```python
from build123d import *

# Parameters (mm, degrees)
F1_DEPTH = 3
F2_DEPTH = 30
F3_W     = 20
F3_H     = 10
F4_DEPTH = 35


with BuildPart() as f1:
    # F0 (on Front) → F1 (new body)
    with BuildSketch(Plane.XZ):
        Polygon((0, 40), (0, 0), (30, 0), (30, 10), (20, 10), (10, 40), align=None)
    extrude(amount=F1_DEPTH)

    # F1_face (on face) → F2 (join)
    with BuildSketch(Plane(origin=(10.666667, -3, 16), x_dir=(1, 0, 0), z_dir=(0, -1, 0))):
        Polygon((-10.666667, 24), (-10.666667, -16), (19.333333, -16), (19.333333, -6), (9.333333, -6), (-0.666667, 24), align=None)
    extrude(amount=F2_DEPTH)

    # F3 (on face) → F4 (cut)
    with BuildSketch(Plane.XY.offset(40)):
        with Locations((20, -15)):
            Rectangle(F3_W, F3_H)
    extrude(amount=-F4_DEPTH, mode=Mode.SUBTRACT)


solid = f1.part
```
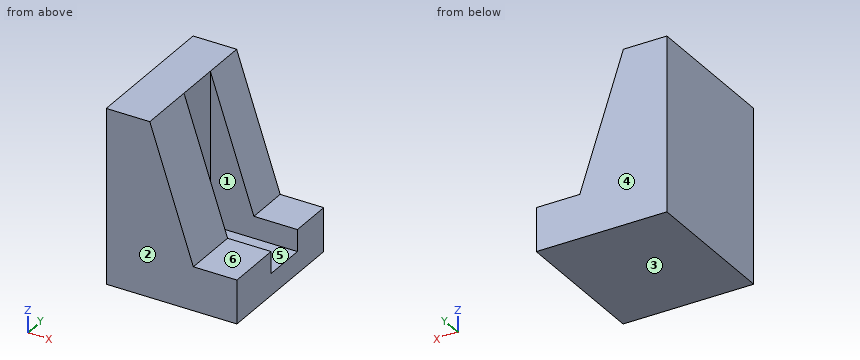
Can you work these out from the model? Positions are in its coordinate system, mm. Face numbers are marked on the shaded views. A direction names the side the tool comes from. Coordinates: 2 decimals unless noted, no trailing zeros. Loops run counter-clockwise (first coordinate to the right, second up) from the corner with the lowest first, then second, coordinate; pieces in that order, holes last. Notation, with made-up numbers: (-16, 27.5) -> (34, 27.5) arc R7 ccw to (34, 34.5) -> close; hole circle Ø1 at (11.25, -28). An arc over 180 degrees is marked (long way). Put each result on its own line as item: value. Start each with the question number.
Q1. For the marked faces 4, 5 and 6, which set-ups out of +Z, -Z, +X, -X, +Y, -Y let a thin tool reach every point of the face, with its end or its side?
Q2. I want a section at B-B (z = 8). Write out the boundary of the cut face in (x, y).
Q3. I want a section at A-A (x = 24.75). Write out the boundary of the cut face in (y, z).
Q4. Thinking about a two-plate mould opening in Y: for the marked faces 1, 2 and 3, which applies, pulls with the +Y half, pulls with the -Y half, needs draft (parallel to the pull), parting line crosses it, or undercut?
Q5. I'm going to push flat-ended pins straight in: P1, Ø5, axis at y = -27.5, z = 14, coming from the +X side; P2, Ø3, axis at x = 22.5, y = -26, coming from the +Z side. Where does each tip first touch, or does it pass through?
Q6. If I drill on line 1 (Y direction, x = 18, z = 11.5); line 2 (Z direction, x = 28.25, y = -8); line 3 (Z direction, x = 20.5, y = -18), over which ranges is the centre line in solid material (lowest first)? Write a range as [from, to].
Q7. I want a section at C-C (y = -10.5). Write out the boundary of the cut face in (x, z).
Taken from the geometry:
1. face 4: +Z, -Z, +X, -X, +Y
1. face 5: +Z, +X
1. face 6: +Z, +X, +Y, -Y
2. outline: (0, -33) -> (30, -33) -> (30, -20) -> (10, -20) -> (10, -10) -> (30, -10) -> (30, 0) -> (0, 0) -> close
3. outline: (-33, 0) -> (0, 0) -> (0, 10) -> (-10, 10) -> (-10, 5) -> (-20, 5) -> (-20, 10) -> (-33, 10) -> close
4. face 1: undercut
4. face 2: pulls with the -Y half
4. face 3: needs draft
5. P1: stops at x = 19.5
5. P2: stops at z = 10
6. line 1: y = [-33, -20], [-10, 0]
6. line 2: z = [0, 10]
6. line 3: z = [0, 5]
7. outline: (0, 0) -> (30, 0) -> (30, 5) -> (10, 5) -> (10, 40) -> (0, 40) -> close
